Part model, mm, in its own coordinate system. A direction names the side the tool comes from. Give positions to 0.01 mm unless a question says otherwise; leave off trailing zeros. Order: outer loops, then holes, each group sorted by start corner. A loop starts at its lowest first (then second) coordinate and runs counter-clockwise, first axis right, second up. Notation, with made-up numbers: (71, 32) -> (76, 32) arc R14 cw to (76, 47) -> close; hole circle Ø11 at (-30.5, 61). An arc over 180 degrees is marked (long way). Write item = value, one per line. Start each with the question number.
(1) Two-plate mould, pull along Z, no slides. Class faces 1 (the flat face through (125, 0, -37)), 2 (the cylindrical face through (46.037, 15.382, -25.223)), 3 (the flat face through (125, 13, -50.8)): pulls with the +Z half, pulls with the -Z half, needs draft (parallel to the pull), parting line crosses it, or undercut.
(2) Saw through at C-C, the plane y = 17.75. State how many separate pieces and enclosed holes the cut face has, then the cut area to 3 significant figures.
(3) Saw through at A-A, the plane x = 127. List the corners of the cut face in (y, z).
(4) Which spindle directions (+Z, -Z, +X, -X, +Y, -Y) get a long thin tool onto all of the face, cutting with end or side? Do faces 4 (the flat face through (80, 15, -9.525)), 5 (the cylindrical face through (239.618, 12.878, -26.847)). Say none if no direction does.
(5) Saw through at B-B, the plane x = 66. List the corners of the cut face in (y, z) (3 decimals), then the cut area to 3 significant figures.
(6) Saw through at D-D, the plane x = 17. List the corners of the cut face in (y, z), then the cut area to 3 significant figures.
(7) Flat gauge pins, fed straight in: pin 1 (20 mm diameter, centred on x = 228.6, z = -25.4, fed in from +Y); pin 2 (16 mm diameter, centred on x = 67.5, z = -28, fed in from +Y). Where does each tip first touch, or does it go through?
(8) Probe line 1 along Z through (x, y) = (97, 8.25) (3 decimals); line 2 along Z through (x, y) = (127.5, 24.25); line 3 along Z through (x, y) = (43.5, 6). List the from-to ranges inside material, lowest first. Write a range as from..to.
from build123d import *

# Parameters (mm, degrees)
SKETCH2_W             = 254
SKETCH2_H             = 50.8
BOSS_EXTRUDE1_DEPTH   = 25.4
SKETCH3_R             = 11.1125
SKETCH3_R_2           = 6.35
CUT_EXTRUDE1_DEPTH    = 261.272549455
F_6_32_TAPPED_HOLE1_D = 3.5052
CUT_EXTRUDE3_DEPTH    = 20.32
CIRPATTERN1_COUNT     = 4
CIRPATTERN2_COUNT     = 4


with BuildPart() as part:
    # Sketch2 → Boss-Extrude1 (new body)
    with BuildSketch(Plane(origin=(0, 0, 0), x_dir=(1, 0, 0), z_dir=(0, 1, 0))):
        with Locations((127, 25.4)):
            Rectangle(SKETCH2_W, SKETCH2_H)
    extrude(amount=BOSS_EXTRUDE1_DEPTH)

    # Sketch3 → Cut-Extrude1 (cut, through all)
    with BuildSketch(Plane(origin=(0, 25.4, 0), x_dir=(1, 0, 0), z_dir=(0, 1, 0))):
        with Locations(Location((25.4, 25.4, 0), (0, 0, 270))):
            Circle(SKETCH3_R)
        with Locations(Location((228.6, 25.4, 0), (0, 0, 270))):
            Circle(SKETCH3_R)
        with Locations(Location((127, 25.4, 0), (0, 0, 270))):
            Circle(SKETCH3_R_2)
    extrude(amount=-CUT_EXTRUDE1_DEPTH, mode=Mode.SUBTRACT)

    # #6-32 Tapped Hole1 (through all)
    with Locations(Plane(origin=(0, 25.4, 0), x_dir=(1, 0, 0), z_dir=(0, 1, 0))):
        with Locations((10.31875, 25.045657608), (243.68125, 25.045657608)):
            f_6_32_tapped_hole1 = Hole(F_6_32_TAPPED_HOLE1_D / 2)

    # Sketch6 → Cut-Extrude3 (cut)
    with BuildSketch(Plane(origin=(0, 25.4, 0), x_dir=(1, 0, 0), z_dir=(0, 1, 0))):
        with BuildLine():
            Line((44.357169653, 41.275), (114.3, 41.275))
            ThreePointArc((114.3, 41.275), (116.658330795, 39.678332318), (116.051724138, 36.895689655))
            ThreePointArc((116.051724138, 36.895689655), (111.125, 25.4), (116.051724138, 13.904310345))
            ThreePointArc((116.051724138, 13.904310345), (116.658330795, 11.121667682), (114.3, 9.525))
            Line((114.3, 9.525), (44.357169653, 9.525))
            ThreePointArc((44.357169653, 9.525), (42.102898213, 10.894589698), (42.279671609, 13.526369863))
            ThreePointArc((42.279671609, 13.526369863), (46.0375, 25.4), (42.279671609, 37.273630137))
            ThreePointArc((42.279671609, 37.273630137), (42.102898213, 39.905410302), (44.357169653, 41.275))
        make_face()
        with BuildLine():
            Line((209.642830347, 41.275), (139.7, 41.275))
            ThreePointArc((139.7, 41.275), (137.341669205, 39.678332318), (137.948275862, 36.895689655))
            ThreePointArc((137.948275862, 36.895689655), (142.875, 25.4), (137.948275862, 13.904310345))
            ThreePointArc((137.948275862, 13.904310345), (137.341669205, 11.121667682), (139.7, 9.525))
            Line((139.7, 9.525), (209.642830347, 9.525))
            ThreePointArc((209.642830347, 9.525), (211.897101787, 10.894589698), (211.720328391, 13.526369863))
            ThreePointArc((211.720328391, 13.526369863), (207.9625, 25.4), (211.720328391, 37.273630137))
            ThreePointArc((211.720328391, 37.273630137), (211.897101787, 39.905410302), (209.642830347, 41.275))
        make_face()
    extrude(amount=-CUT_EXTRUDE3_DEPTH, mode=Mode.SUBTRACT)

    # CirPattern1: #6-32 Tapped Hole1 ×4 about axis
    cirpattern1_axis = Axis((25.4, 0, -25.4), (0, 1, 0))
    for i in range(1, CIRPATTERN1_COUNT):
        add(f_6_32_tapped_hole1.rotate(cirpattern1_axis, i * 360 / CIRPATTERN1_COUNT), mode=Mode.SUBTRACT)

    # CirPattern2: #6-32 Tapped Hole1 ×4 about axis
    cirpattern2_axis = Axis((228.6, 0, -25.4), (0, 1, 0))
    for i in range(1, CIRPATTERN2_COUNT):
        add(f_6_32_tapped_hole1.rotate(cirpattern2_axis, i * 360 / CIRPATTERN2_COUNT), mode=Mode.SUBTRACT)


solid = part.part
Results list:
q1.face_1 = needs draft
q1.face_2 = undercut
q1.face_3 = pulls with the -Z half
q2.separate_pieces = 1
q2.enclosed_holes = 13
q2.area = 7,510 mm^2
q3.outline = (0, -50.8) -> (25.4, -50.8) -> (25.4, -31.75) -> (0, -31.75) -> close; (0, -19.05) -> (25.4, -19.05) -> (25.4, 0) -> (0, 0) -> close
q4.face_4 = +Y
q4.face_5 = +Y, -Y
q5.outline = (0, -50.8) -> (25.4, -50.8) -> (25.4, -41.275) -> (5.08, -41.275) -> (5.08, -9.525) -> (25.4, -9.525) -> (25.4, 0) -> (0, 0) -> close
q5.area = 645 mm^2
q6.outline = (0, -50.8) -> (25.4, -50.8) -> (25.4, -32.68) -> (0, -32.68) -> close; (0, -18.12) -> (25.4, -18.12) -> (25.4, 0) -> (0, 0) -> close
q6.area = 921 mm^2
q7.pin_1 = through
q7.pin_2 = 5.08
q8.line_1 = -50.8..-41.275, -9.525..0
q8.line_2 = -50.8..-31.73, -19.07..0
q8.line_3 = -50.8..-41.13, -35.31..-15.49, -9.67..0
